Could you check a few things on this drawing? It's one solid part, dimensions in mm from its lowest x, y, z. A direction names the side the tool comes from. Give positions to 0.01 mm unless a question says otherwise; leave off trailing zeros. Loops run counter-clockwise (first coordinate to the right, second up) from the corner with the lowest first, then second, coordinate; pieces in that order, holes last. Notation, with made-up numbers: (52.25, 43) -> (110.25, 43) arc R36 cw to (110.25, 78) -> close; hole circle Ø1 at (83.5, 4). An arc over 180 degrees is marked (long way). Use CSV: the item, a comma, the result in double quotes.
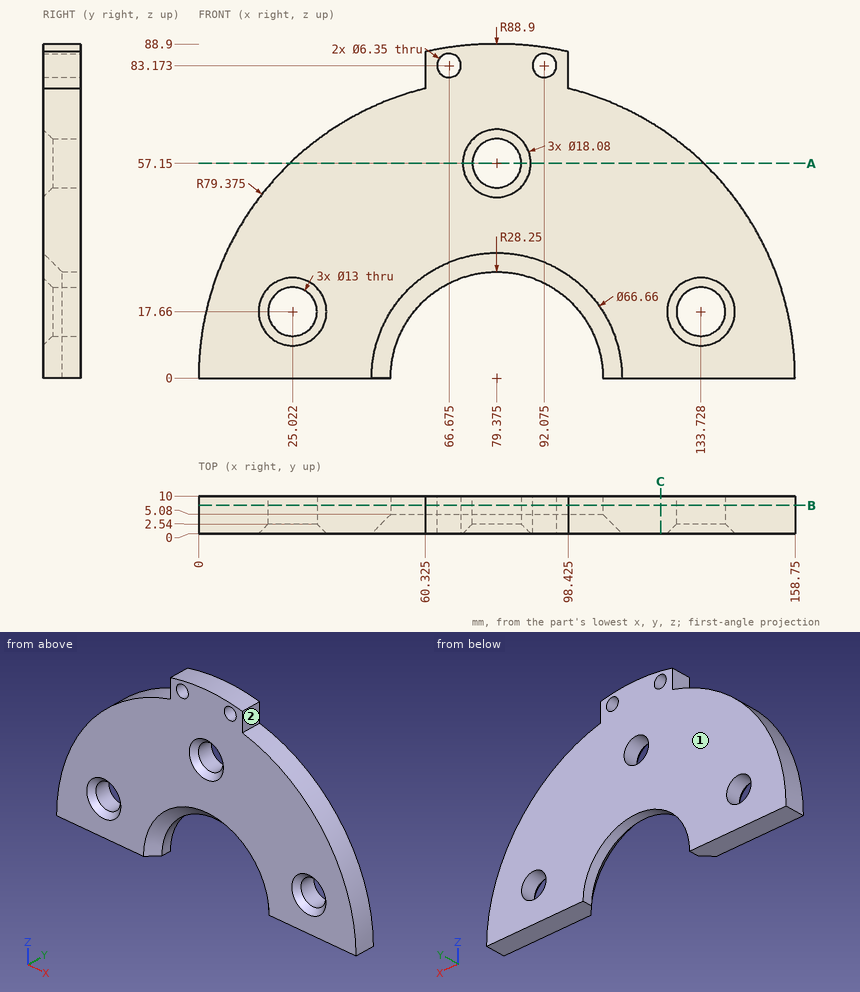
(1) Will these pins go through, and if not, where does the flat tip stop? pin 1 Ø3 at (y, z) = (6, 82) entering from +X (1 decimal); pin 2 Ø11.5 at (x, z) = (79.375, 57.15) entering from -Y; pin 3 Ø5 at (y, z) = (5, 80) entering from -X (1 decimal); pin 4 Ø1 at (x, z) = (50, 72) entering from -Y.
Answer sheet:
pin 1,"stops at x = 98.4"
pin 2,"passes through"
pin 3,"stops at x = 60.3"
pin 4,"stops at y = 0"
(2) If I drill on L1, parallel to X at y = 5, z = 84 (1 decimal); L2, parallel to X at y = 9, z = 16.5 (1 decimal); L3, parallel to X at y = 9.25, z = 63 (1 decimal), over which ranges is the centre line in solid material (lowest first)? Write a range as from..to.
Answer sheet:
L1,"x = 60.3..63.6, 69.7..89, 95.1..98.4"
L2,"x = 1.7..18.6, 31.4..56.4, 102.3..127.3, 140.1..157"
L3,"x = 31.1..76.5, 82.2..127.7"
(3) Which directions (+Z, -Z, +X, -X, +Y, -Y) give clear straight access to the entire face, cutting with the end or side of a thin tool? Please do the marked faces 1 and 2.
Answer sheet:
face 1,"+Z, -Z, +X, -X, +Y"
face 2,"+Z, +X, +Y, -Y"
(4) If we section it at B-B, the plane y = 7.5: Give the number of separate pieces and of enclosed holes in the cut face, then the cut area to 3 significant figures.
Answer sheet:
separate pieces,"1"
enclosed holes,"5"
area,"8,550 mm2"
(5) If we section it at A-A, the plane z = 57.15: Write out the boundary of the cut face in (x, y) (1 decimal).
Answer sheet:
outline,"(24.3, 0) -> (70.3, 0) -> (72.9, 2.5) -> (72.9, 10) -> (24.3, 10) -> close; (85.9, 2.5) -> (88.4, 0) -> (134.5, 0) -> (134.5, 10) -> (85.9, 10) -> close"
(6) If we section it at C-C, the plane x = 123: Write out the boundary of the cut face in (y, z), then the cut area to 3 significant figures.
Answer sheet:
outline,"(0, 0) -> (10, 0) -> (10, 66.31) -> (0, 66.31) -> close"
area,"663 mm2"
